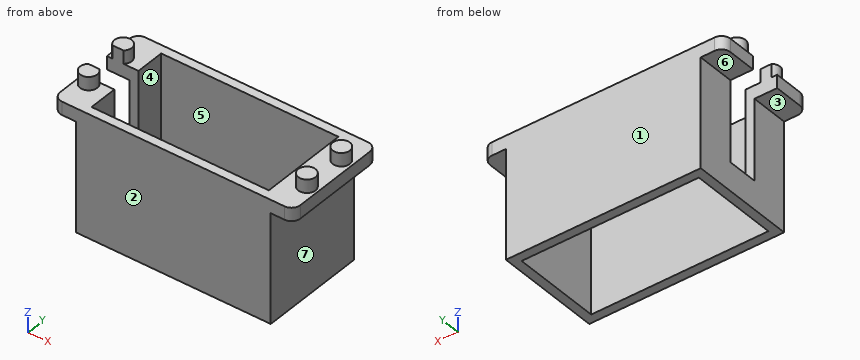
from build123d import *

# Parameters (mm, degrees)
BOSS_EXTRU_1_DEPTH = 27.8
ESQUISSE3_W        = 2
ESQUISSE3_H        = 7
BOSS_EXTRU_2_DEPTH = 6.44
BOSS_EXTRU_3_DEPTH = 3
ESQUISSE7_R        = 1.95
BOSS_EXTRU_4_DEPTH = 3


with BuildPart() as part:
    # Esquisse1 → Boss.-Extru.1 (new body)
    with BuildSketch(Plane.XY):
        Polygon((-2, 22.2), (-2, 13.6), (0, 13.6), (0, 20.2), (40.2, 20.2), (40.2, 0), (0, 0), (0, 6.6), (-2, 6.6), (-2, -2), (42.2, -2), (42.2, 22.2), align=None)
    extrude(amount=BOSS_EXTRU_1_DEPTH)

    # Esquisse3 → Boss.-Extru.2 (add)
    with BuildSketch(Plane(origin=(0, 0, 0), x_dir=(-1, 0, 0), z_dir=(0, 0, -1))):
        with Locations((1, 10.1)):
            Rectangle(ESQUISSE3_W, ESQUISSE3_H)
    extrude(amount=-BOSS_EXTRU_2_DEPTH)

    # Esquisse5 → Boss.-Extru.3 (add)
    with BuildSketch(Plane.XY.offset(27.8)):
        with BuildLine():
            Line((-2, 13.6), (-2, 22.2))
            Line((-2, 22.2), (-5.15, 22.2))
            ThreePointArc((-5.15, 22.2), (-6.564213562, 21.614213562), (-7.15, 20.2))
            Line((-7.15, 20.2), (-7.15, 13.6))
            Line((-7.15, 13.6), (-2, 13.6))
        make_face()
        with BuildLine():
            Line((-2, -2), (-2, 6.6))
            Line((-2, 6.6), (-7.15, 6.6))
            Line((-7.15, 6.6), (-7.15, 0))
            ThreePointArc((-7.15, 0), (-6.564213562, -1.414213562), (-5.15, -2))
            Line((-5.15, -2), (-2, -2))
        make_face()
        with BuildLine():
            Line((42.2, -2), (45.35, -2))
            ThreePointArc((45.35, -2), (46.764213562, -1.414213562), (47.35, 0))
            Line((47.35, 0), (47.35, 20.2))
            ThreePointArc((47.35, 20.2), (46.764213562, 21.614213562), (45.35, 22.2))
            Line((45.35, 22.2), (42.2, 22.2))
            Line((42.2, 22.2), (42.2, -2))
        make_face()
    extrude(amount=-BOSS_EXTRU_3_DEPTH)

    # Esquisse7 → Boss.-Extru.4 (add)
    with BuildSketch(Plane.XY.offset(27.8)):
        with Locations(Location((44.85, 5.1, 0), (0, 0, 180))):
            Circle(ESQUISSE7_R)
        with Locations(Location((44.85, 15.1, 0), (0, 0, 180))):
            Circle(ESQUISSE7_R)
        with BuildLine():
            Line((-5.895993579, 13.6), (-3.404006421, 13.6))
            ThreePointArc((-3.404006421, 13.6), (-4.65, 17.05), (-5.895993579, 13.6))
        make_face()
        with BuildLine():
            Line((-5.895993579, 6.6), (-3.404006421, 6.6))
            ThreePointArc((-3.404006421, 6.6), (-4.65, 3.15), (-5.895993579, 6.6))
        make_face()
    extrude(amount=BOSS_EXTRU_4_DEPTH)


solid = part.part
The listing builds one solid part. Answer for the finished solid, in the listing's coordinates (mm). Face numbers are marked on the shaded views. A direction names the side the tool comes from. Round coordinates to 2 decimals unless told otherwise and drop trailing zeros. Order: outer loops, then holes, each group sorted by start corner. A loop starts at its lowest first (then second) coordinate and runs counter-clockwise, first axis right, second up. Notation, with made-up numbers: (-24.75, 36) -> (9.25, 36) arc R18 ccw to (9.25, 59) -> close; hole circle Ø10 at (-9.5, -33). An arc over 180 degrees is marked (long way). One line per item, written item: value.
Item 1: Find section B-B, the plane z = 3.5. Give the vertices of the cut face in (x, y).
Taken from the geometry:
outline: (-2, -2) -> (42.2, -2) -> (42.2, 22.2) -> (-2, 22.2) -> close; hole (0, 0) -> (40.2, 0) -> (40.2, 20.2) -> (0, 20.2) -> close
Item 2: Find section C-C, the plane x = 7. Give the vertices of the cut face in (y, z).
Taken from the geometry:
outline: (-2, 0) -> (0, 0) -> (0, 27.8) -> (-2, 27.8) -> close; (20.2, 0) -> (22.2, 0) -> (22.2, 27.8) -> (20.2, 27.8) -> close
Item 3: Find section A-A, the plane y = 5.1. Give the vertices of the cut face in (x, z).
Taken from the geometry:
outline: (-7.15, 24.8) -> (-2, 24.8) -> (-2, 0) -> (0, 0) -> (0, 27.8) -> (-2.7, 27.8) -> (-2.7, 30.8) -> (-6.6, 30.8) -> (-6.6, 27.8) -> (-7.15, 27.8) -> close; (40.2, 0) -> (42.2, 0) -> (42.2, 24.8) -> (47.35, 24.8) -> (47.35, 27.8) -> (46.8, 27.8) -> (46.8, 30.8) -> (42.9, 30.8) -> (42.9, 27.8) -> (40.2, 27.8) -> close
Item 4: For the marked faces 5, 6 and 7, determine the directions among +Z, -Z, +X, -X, +Y, -Y from which every point of the face is accessible in a straight line to the end or side of a thin tool.
Taken from the geometry:
face 5: +Z, -Z
face 6: -Z, -X, +Y, -Y
face 7: -Z, +X, +Y, -Y
Item 5: Find section D-D, the plane z = 24. Give the vertices of the cut face in (x, y).
Taken from the geometry:
outline: (-2, -2) -> (42.2, -2) -> (42.2, 22.2) -> (-2, 22.2) -> (-2, 13.6) -> (0, 13.6) -> (0, 20.2) -> (40.2, 20.2) -> (40.2, 0) -> (0, 0) -> (0, 6.6) -> (-2, 6.6) -> close
Item 6: Given P1, Ø3, axis at y = 7.5, z = 19, coming from the -X side; P2, Ø6, axis at y = 8, z = 14.5, coming from the +X side; P3, Ø5.5, axis at x = -5.5, y = 3, coming from the -Z side; P4, Ø12, axis at x = 17.5, y = 7.5, coming from the +Z side, each flat-ended and moving along its own axis, determine where each tip first touches the part or whether it passes through.
Taken from the geometry:
P1: stops at x = -2
P2: stops at x = 42.2
P3: stops at z = 24.8
P4: passes through
Item 7: For a pull along Y with two mould halves and no side action, classify the marked faces 1, 2, 3 and 4 as released by +Y, released by -Y, zero draft, split by the parting line, or undercut.
Taken from the geometry:
face 1: released by +Y
face 2: released by -Y
face 3: zero draft
face 4: undercut
Item 8: Straight lines are drawn through the part: L1, parallel to Y at x = 29, z = 7; L2, parallel to X at y = 17, z = 21; L3, parallel to X at y = 12, z = 7. For each, find the intervals that lie inside material, in ascending order.
Taken from the geometry:
L1: y = -2 to 0, 20.2 to 22.2
L2: x = -2 to 0, 40.2 to 42.2
L3: x = 40.2 to 42.2
